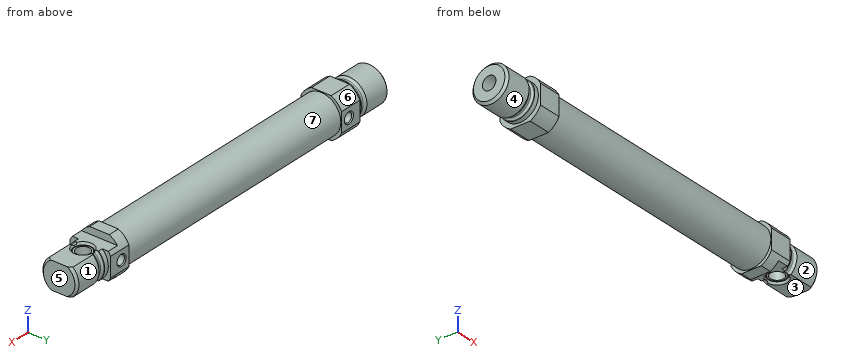
from build123d import *

# Parameters (mm, degrees)
BOSS_EXTRUDE1_DEPTH     = 10
SKETCH3_W               = 116
SKETCH3_H               = 8.65
SKETCH4_W               = 18
SKETCH4_H               = 18
BOSS_EXTRUDE2_DEPTH     = 10
SKETCH5_W               = 10
SKETCH5_H               = 10
CUT_EXTRUDE1_DEPTH      = 10
CUT_EXTRUDE1_DEPTH_BACK = 10
HOLE1_D                 = 4.134
HOLE1_DEPTH             = 9
HOLE1_CSINK_D           = 5
HOLE1_CSINK_ANGLE       = 90
HOLE2_D                 = 4.134
HOLE2_DEPTH             = 11
HOLE2_CSINK_D           = 5
HOLE2_CSINK_ANGLE       = 90
HOLE2_TIP               = 1.193383006


with BuildPart() as part:
    # Sketch1 → Revolve1 (revolve)
    with BuildSketch(Plane.XY):
        with BuildLine():
            Line((0, 0), (0, 7))
            Line((0, 7), (1, 8))
            Line((1, 8), (11.95, 8))
            Line((11.95, 8), (12.865685425, 7.084314575))
            ThreePointArc((12.865685425, 7.084314575), (13.125224104, 6.910896374), (13.43137085, 6.85))
            Line((13.43137085, 6.85), (14.2, 6.85))
            ThreePointArc((14.2, 6.85), (14.765685425, 7.084314575), (15, 7.65))
            Line((15, 7.65), (15, 8))
            Line((15, 8), (17, 8))
            Line((17, 8), (17, 0))
            Line((17, 0), (0, 0))
        make_face()
    revolve(axis=Axis((17, 0, 0), (-1, 0, 0)))

    # Sketch2 → Boss-Extrude1 (add)
    with BuildSketch(Plane(origin=(17, 0, 0), x_dir=(0, 0, -1), z_dir=(1, 0, 0))):
        with BuildLine():
            Line((-4.358898944, -9), (4.358898944, -9))
            ThreePointArc((4.358898944, -9), (7.071067812, -7.071067812), (9, -4.358898944))
            Line((9, -4.358898944), (9, 4.358898944))
            ThreePointArc((9, 4.358898944), (7.071067812, 7.071067812), (4.358898944, 9))
            Line((4.358898944, 9), (-4.358898944, 9))
            ThreePointArc((-4.358898944, 9), (-7.071067812, 7.071067812), (-9, 4.358898944))
            Line((-9, 4.358898944), (-9, -4.358898944))
            ThreePointArc((-9, -4.358898944), (-7.071067812, -7.071067812), (-4.358898944, -9))
        make_face()
    extrude(amount=BOSS_EXTRUDE1_DEPTH)

    # Sketch3 → Revolve2 (revolve)
    with BuildSketch(Plane.XY):
        with Locations((85, 4.325)):
            Rectangle(SKETCH3_W, SKETCH3_H)
    revolve(axis=Axis((143, 0, 0), (-1, 0, 0)))

    # Sketch4 → Boss-Extrude2 (add)
    with BuildSketch(Plane(origin=(143, 0, 0), x_dir=(0, 0, -1), z_dir=(1, 0, 0))):
        Rectangle(SKETCH4_W, SKETCH4_H)
    extrude(amount=BOSS_EXTRUDE2_DEPTH)

    # Sketch5 → Cut-Revolve1 (revolve, cut)
    with BuildSketch(Plane.XY):
        with Locations((148, 15)):
            Rectangle(SKETCH5_W, SKETCH5_H)
    revolve(axis=Axis((153, 0, 0), (-1, 0, 0)), mode=Mode.SUBTRACT)

    # Sketch6 → Revolve3 (revolve)
    with BuildSketch(Plane.XY):
        with BuildLine():
            Line((153, 0), (153, 8))
            Line((153, 8), (155, 8))
            Line((155, 8), (155, 7.65))
            ThreePointArc((155, 7.65), (155.234314575, 7.084314575), (155.8, 6.85))
            Line((155.8, 6.85), (156.56862915, 6.85))
            ThreePointArc((156.56862915, 6.85), (156.874775896, 6.910896374), (157.134314575, 7.084314575))
            Line((157.134314575, 7.084314575), (158.05, 8))
            Line((158.05, 8), (169, 8))
            Line((169, 8), (170, 7))
            Line((170, 7), (170, 0))
            Line((170, 0), (153, 0))
        make_face()
    revolve(axis=Axis((170, 0, 0), (-1, 0, 0)))

    # Sketch7 → Cut-Extrude1 (cut, two sides)
    with BuildSketch(Plane(origin=(0, 0, 0), x_dir=(1, 0, 0), z_dir=(0, 1, 0))) as cut_extrude1_sk:
        Polygon((148, 18), (148, 6), (170, 6), (170, -6), (148, -6), (148, -18), (182, -18), (182, 18), align=None)
    extrude(amount=CUT_EXTRUDE1_DEPTH, mode=Mode.SUBTRACT)
    extrude(cut_extrude1_sk.sketch, amount=-CUT_EXTRUDE1_DEPTH_BACK, mode=Mode.SUBTRACT)

    # Sketch8 → Cut-Revolve2 (revolve, cut)
    with BuildSketch(Plane(origin=(157, 0, 0), x_dir=(0, 0, -1), z_dir=(1, 0, 0))):
        Polygon((-6.2, 0), (-6.2, 4.692820323), (-5, 4), (-4.5, 4), (-5, 3.711324865), (-5, 3), (5, 3), (5, 3.711324865), (4.5, 4), (5, 4), (6.2, 4.692820323), (6.2, 0), align=None)
    revolve(axis=Axis((157, 0, -5), (0, 0, 1)), mode=Mode.SUBTRACT)

    # Hole1
    with Locations(Plane(origin=(0, 9, 0), x_dir=(1, 0, 0), z_dir=(0, 1, 0))):
        with Locations((23, 0)):
            CounterSinkHole(HOLE1_D / 2, HOLE1_CSINK_D / 2, depth=HOLE1_DEPTH, counter_sink_angle=HOLE1_CSINK_ANGLE)

    # Hole2
    with Locations(Plane(origin=(0, 9, 0), x_dir=(1, 0, 0), z_dir=(0, 1, 0))):
        with Locations((147, 0)):
            CounterSinkHole(HOLE2_D / 2, HOLE2_CSINK_D / 2, depth=HOLE2_DEPTH, counter_sink_angle=HOLE2_CSINK_ANGLE)
            with Locations((0, 0, -(HOLE2_DEPTH + HOLE2_TIP / 2))):  # 120° drill point
                Cone(0, HOLE2_D / 2, HOLE2_TIP, mode=Mode.SUBTRACT)

    # Sketch13 → Cut-Revolve3 (revolve, cut)
    with BuildSketch(Plane.XY):
        Polygon((-5, 0), (-5, 3), (41.2, 3), (41.2, 8), (125.2, 8), (125.2, 0), align=None)
    revolve(axis=Axis((125.2, 0, 0), (-1, 0, 0)), mode=Mode.SUBTRACT)


solid = part.part
The model under review builds one solid part; all positions refer to its coordinate system, in mm. Face numbers are marked on the shaded views. A direction names the side the tool comes from. Give positions to 0.01 mm unless a question says otherwise; leave off trailing zeros. Order: outer loops, then holes, each group sorted by start corner. A loop starts at its lowest first (then second) coordinate and runs counter-clockwise, first axis right, second up. Notation, with made-up numbers: M 30.25,-31 L 80.25,-31 A10 ccw 80.25,-17 Z; hole C -8.75,-9.75 d11. An arc over 180 degrees is marked long. Answer in a Markdown table with one row per item. Add a question column.
1. Machinability: for the marked faces 1, 2, 3 and 4, which of the approach directions +Z, -Z, +X, -X, +Y, -Y give a long, thin tool a straight path to every point of the face, cutting with its end or side? Answer none if there is none.
2. Add section B-B on x = 23. State the section outline as (y, z) points.
3. To check wall thickness, follow line 1 along X through (y, z) = (0, 4.95); line 2 along Y through (x, z) = (15.5, 0); line 3 along Y through (x, z) = (49, 6.25). State the ranges of each line that lie inside material, in increasing order.
4. For pin 1 Ø5.5 at (y, z) = (-0.5, -2.5) entering from -X; pin 2 Ø1 at (x, z) = (35.5, -3) entering from +Y; pin 3 Ø10.5 at (x, y) = (157, 0) entering from -Z; pin 4 Ø10 at (x, y) = (103.5, 7) entering from -Z, all flat-tipped, find the tip position at first contact; note any pin that passes through.
5. Add section A-A on y = 0. Count the separate pieces of the cut face and the enclosed holes in it, plus the area to 3 significant figures.
6. Mouldability with a two-part tool opening along X and no side actions: class the marked faces 5, 6 and 7 as released by +X, released by -X, zero draft, split by the parting line, or undercut.
The answers:
| question | item | result |
|---|---|---|
| 1 | face 1 | +X, +Y |
| 1 | face 2 | +X, -Y |
| 1 | face 3 | -Z, +X, +Y, -Y |
| 1 | face 4 | -X |
| 2 | outline | M -9,-4.36 A10 ccw -4.36,-9 L 4.36,-9 A10 ccw 9,-4.36 L 9,-2.5 L 8.57,-2.07 L 2.17,-2.07 A3 cw long 2.17,2.07 L 8.57,2.07 L 9,2.5 L 9,4.36 A10 ccw 4.36,9 L -4.36,9 A10 ccw -9,4.36 Z |
| 3 | line 1 | 0 to 41.2, 125.2 to 153, 153.26 to 154, 160 to 160.74, 161 to 170 |
| 3 | line 2 | -8 to -3, 3 to 8 |
| 3 | line 3 | -5.98 to -4.99, 4.99 to 5.98 |
| 4 | pin 1 | x = 0 |
| 4 | pin 2 | y = 8.28 |
| 4 | pin 3 | z = -6 |
| 4 | pin 4 | z = -8.42 |
| 5 | separate pieces | 2 |
| 5 | enclosed holes | 1 |
| 5 | area | 1,120 mm2 |
| 6 | face 5 | released by +X |
| 6 | face 6 | zero draft |
| 6 | face 7 | undercut |
